```python
from build123d import *

# Parameters (mm, degrees)
SKETCH1_R           = 35
BOSS_EXTRUDE1_DEPTH = 10
CUT_EXTRUDE1_REACH  = 52.498
SKETCH2_R           = 2
CIRPATTERN1_COUNT   = 4
SKETCH5_W           = 10
SKETCH5_H           = 16.60119737
CUT_EXTRUDE2_DEPTH  = 51.497524692
CIRPATTERN2_COUNT   = 3
SKETCH6_R           = 20
CUT_EXTRUDE3_DEPTH  = 6.5


with BuildPart() as part:
    # Sketch1 → Boss-Extrude1 (new body)
    with BuildSketch(Plane(origin=(0, 0, 0), x_dir=(1, 0, 0), z_dir=(0, 1, 0))):
        with Locations(Location((0, 0, 0), (0, 0, 270))):
            Circle(SKETCH1_R)
    extrude(amount=BOSS_EXTRUDE1_DEPTH)

    # Sketch2 → Cut-Extrude1 (cut, up to next)
    with BuildSketch(Plane(origin=(0, 10, 0), x_dir=(1, 0, 0), z_dir=(0, 1, 0)), mode=Mode.PRIVATE) as cut_extrude1_sk1:
        with Locations(Location((0, 15, 0), (0, 0, 270))):
            Circle(SKETCH2_R)
    cut_extrude1_tool1 = extrude(cut_extrude1_sk1.sketch, amount=-CUT_EXTRUDE1_REACH, mode=Mode.PRIVATE) & part.part
    cut_extrude1 = cut_extrude1_tool1.solids().sort_by_distance((0, 10, -15))[0]
    add(cut_extrude1, mode=Mode.SUBTRACT)

    # CirPattern1: Cut-Extrude1 ×4 about axis
    cirpattern1_axis = Axis((0, 0, 0), (0, 1, 0))
    for i in range(1, CIRPATTERN1_COUNT):
        add(cut_extrude1.rotate(cirpattern1_axis, i * 360 / CIRPATTERN1_COUNT), mode=Mode.SUBTRACT)

    # Sketch5 → Cut-Extrude2 (cut, symmetric)
    with BuildSketch(Plane.XY):
        with Locations((0, 11.800598685)):
            Rectangle(SKETCH5_W, SKETCH5_H)
    cut_extrude2 = extrude(amount=CUT_EXTRUDE2_DEPTH, both=True, mode=Mode.SUBTRACT)

    # CirPattern2: Cut-Extrude2 ×3 about axis
    cirpattern2_axis = Axis((0, 0, 0), (0, 1, 0))
    for i in range(1, CIRPATTERN2_COUNT):
        add(cut_extrude2.rotate(cirpattern2_axis, i * 360 / CIRPATTERN2_COUNT), mode=Mode.SUBTRACT)

    # Sketch6 → Cut-Extrude3 (cut)
    with BuildSketch(Plane(origin=(0, 10, 0), x_dir=(1, 0, 0), z_dir=(0, 1, 0))):
        Circle(SKETCH6_R)
    extrude(amount=-CUT_EXTRUDE3_DEPTH, mode=Mode.SUBTRACT)


solid = part.part
```
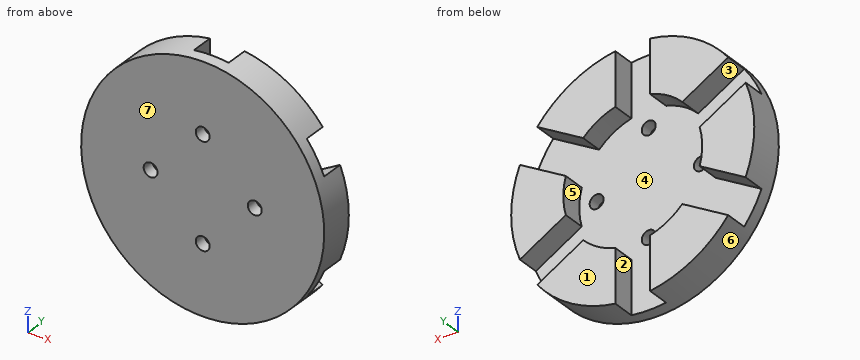
Here's how the part is built. I have some questions about the finished solid (model axes, mm). Face numbers are marked on the shaded views. A direction names the side the tool comes from. Coordinates: 2 decimals unless noted, no trailing zeros. Order: outer loops, then holes, each group sorted by start corner. A loop starts at its lowest first (then second) coordinate and runs counter-clockwise, first axis right, second up. Notation, with made-up numbers: (-3, 31.25) - (23, 31.25) arc R21 ccw to (23, 66.25) - close; hole circle Ø4 at (7, -26.5). An arc over 180 degrees is marked (long way). One line per question, with ' | ' between items. Start each with the question number.
1. If we mould it in two halves opening along X, with no side actions, what happens to the marked faces 5, 6 and 7? For each: released by +X, released by -X, zero draft, split by the parting line, or undercut.
2. Please list where these lines run through material, in increasing order: line 1 along Z through (x, y) = (21, 7.75); line 2 along Y through (x, z) = (-13.5, 2.5); line 3 along X through (y, z) = (5, 21.5). Write a range as [from, to].
3. If we section it at B-B (y = 8.5): Write out the boundary of the cut face in (x, z), and give its area (3 significant figures).
4. Which directions (+Z, -Z, +X, -X, +Y, -Y) give clear straight access to the entire face, cutting with the end or side of a thin tool? Please do the marked faces 1, 2, 3 and 4.
5. I'm going to push flat-ended pins straight in: pin 1 Ø6.5 at (x, z) = (15, 0) entering from +Y; pin 2 Ø3 at (y, z) = (7, -2.5) entering from +X; pin 3 Ø2 at (y, z) = (6, -29) entering from +X; pin 4 Ø3 at (x, z) = (-15, 0) entering from -Y. Where does each tip first touch, or does it pass through?
6. If we section it at A-A (z = 0): Write out the boundary of the cut face in (x, y), and give its area (3 significant figures).
7. If we section it at C-C (x = 0): Write out the boundary of the cut face in (y, z), and give its area (3 significant figures).
8. If we section it at D-D (z = -15): Write out the boundary of the cut face in (x, y).
Model answer:
1) face 5: undercut | face 6: split by the parting line | face 7: zero draft
2) line 1: z = [-28, -17.9], [-6.35, 6.35], [17.9, 28] | line 2: y = [0, 3.5] | line 3: x = [-27.24, -5], [5, 27.24]
3) outline: (-32.5, -12.99) - (-19.27, -5.35) arc R20 cw to (-19.27, 5.35) - (-32.5, 12.99) arc R35 ccw to start; (-27.5, -21.65) arc R35 ccw to (-5, -34.64) - (-5, -19.36) arc R20 cw to (-14.27, -14.01) - close; (-27.5, 21.65) - (-14.27, 14.01) arc R20 cw to (-5, 19.36) - (-5, 34.64) arc R35 ccw to start; (5, -34.64) arc R35 ccw to (27.5, -21.65) - (14.27, -14.01) arc R20 cw to (5, -19.36) - close; (5, 19.36) arc R20 cw to (14.27, 14.01) - (27.5, 21.65) arc R35 ccw to (5, 34.64) - close; (19.27, -5.35) - (32.5, -12.99) arc R35 ccw to (32.5, 12.99) - (19.27, 5.35) arc R20 cw to start | area: 1,690 mm²
4) face 1: +Z, -Z, +X, -X, +Y | face 2: +Z, -Z, +Y | face 3: -X, +Y | face 4: +Y
5) pin 1: stops at y = 3.5 | pin 2: stops at x = 34.99 | pin 3: stops at x = 21 | pin 4: passes through
6) outline: (-35, 0) - (-17, 0) - (-17, 3.5) - (-20, 3.5) - (-20, 10) - (-35, 10) - close; (-13, 0) - (13, 0) - (13, 3.5) - (-13, 3.5) - close; (17, 0) - (35, 0) - (35, 10) - (20, 10) - (20, 3.5) - (17, 3.5) - close | area: 412 mm²
7) outline: (0, -35) - (3.5, -35) - (3.5, -17) - (0, -17) - close; (0, -13) - (3.5, -13) - (3.5, 13) - (0, 13) - close; (0, 17) - (3.5, 17) - (3.5, 35) - (0, 35) - close | area: 217 mm²
8) outline: (-31.62, 0) - (-2, 0) - (-2, 3.5) - (-13.23, 3.5) - (-13.23, 10) - (-15.98, 10) - (-15.98, 3.5) - (-31.62, 3.5) - close; (2, 0) - (31.62, 0) - (31.62, 3.5) - (15.98, 3.5) - (15.98, 10) - (13.23, 10) - (13.23, 3.5) - (2, 3.5) - close
